Verification items for the finished model (mm, model axes). A direction names the side the tool comes from. Give positions to 0.01 mm unless a question says otherwise; leave off trailing zeros. Write each loop counter-clockwise with the first axis right and the second up, starting at its lowest first coordinate (ties: lowest second). Pieces come first, ordered by that corner, then holes. Notation, with made-up numbers: (-7, 89.25) -> (29, 89.25) arc R20 ccw to (29, 101.25) -> close; hole circle Ø1 at (-26.75, 72.25). An arc over 180 degrees is marked (long way). Write item = value, one per line.
from build123d import *

# Parameters (mm, degrees)
BOSS_EXTRUDE1_DEPTH = 3
SKETCH3_R           = 5.053902861
SKETCH3_R_2         = 2.749769833
BOSS_EXTRUDE3_DEPTH = 3
CUT_EXTRUDE1_DEPTH  = 3
SKETCH5_W           = 3
SKETCH5_H           = 8
CUT_EXTRUDE2_DEPTH  = 3


with BuildPart() as part:
    # Sketch1 → Boss-Extrude1 (new body)
    with BuildSketch(Plane.XY):
        with BuildLine():
            Line((-7, -3), (3, -3))
            Line((3, -3), (3, 0))
            Line((3, 0), (23, 0))
            Line((23, 0), (23, -3))
            Line((23, -3), (33, -3))
            Line((33, -3), (33, 0))
            Line((33, 0), (51.582575695, 0))
            ThreePointArc((51.582575695, 0), (51.894531565, 0.978451782), (52, 2))
            Line((52, 2), (52, 19.311841589))
            ThreePointArc((52, 19.311841589), (51.894531565, 20.333389808), (51.582575695, 21.311841589))
            Line((51.582575695, 21.311841589), (33, 21.311841589))
            Line((33, 21.311841589), (33, 24.311841589))
            Line((33, 24.311841589), (23, 24.311841589))
            Line((23, 24.311841589), (23, 21.311841589))
            Line((23, 21.311841589), (3, 21.311841589))
            Line((3, 21.311841589), (3, 24.311841589))
            Line((3, 24.311841589), (-7, 24.311841589))
            Line((-7, 24.311841589), (-7, 21.311841589))
            Line((-7, 21.311841589), (-25.582575695, 21.311841589))
            ThreePointArc((-25.582575695, 21.311841589), (-25.894531565, 20.333389808), (-26, 19.311841589))
            Line((-26, 19.311841589), (-26, 2))
            ThreePointArc((-26, 2), (-25.894531565, 0.978451782), (-25.582575695, 0))
            Line((-25.582575695, 0), (-7, 0))
            Line((-7, 0), (-7, -3))
        make_face()
    extrude(amount=BOSS_EXTRUDE1_DEPTH)

    # Sketch3 → Boss-Extrude3 (add)
    with BuildSketch(Plane(origin=(0, 0, 0), x_dir=(-1, 0, 0), z_dir=(0, 0, -1))):
        with Locations((20.946097139, 22.811841589)):
            Circle(SKETCH3_R)
        with Locations((20.946097139, 22.811841589)):
            Circle(SKETCH3_R_2, mode=Mode.SUBTRACT)
    extrude(amount=-BOSS_EXTRUDE3_DEPTH)

    # Sketch4 → Cut-Extrude1 (cut)
    with BuildSketch(Plane(origin=(0, 0, 0), x_dir=(-1, 0, 0), z_dir=(0, 0, -1))):
        with BuildLine():
            Line((23.250708633, 21.311841589), (18.641485645, 21.311841589))
            ThreePointArc((18.641485645, 21.311841589), (20.946097139, 20.062071756), (23.250708633, 21.311841589))
        make_face()
    extrude(amount=-CUT_EXTRUDE1_DEPTH, mode=Mode.SUBTRACT)

    # Sketch5 → Cut-Extrude2 (cut)
    with BuildSketch(Plane(origin=(0, 0, 0), x_dir=(-1, 0, 0), z_dir=(0, 0, -1))):
        with Locations((24.5, 10.655920795)):
            Rectangle(SKETCH5_W, SKETCH5_H)
        with Locations((-50.5, 10.655920795)):
            Rectangle(SKETCH5_W, SKETCH5_H)
    extrude(amount=-CUT_EXTRUDE2_DEPTH, mode=Mode.SUBTRACT)


solid = part.part
Item 1: Set-up check for faces 1 (the flat face through (51, 6.656, 1)), 2 (the flat face through (23, -1, 1)), 3 (the flat face through (-7, -1, 1)), 4 (the flat face through (42, 0, 1)): record each of +Z, -Z, +X, -X, +Y, -Y from which the full face is reachable in a straight line by a thin tool's end or side.
Response values:
face_1 = +Z, -Z, +X
face_2 = +Z, -Z, -Y
face_3 = +Z, -Z, -X, -Y
face_4 = +Z, -Z, +X, -Y
Item 2: Material ranges on line 1 (X direction, y = 22.5, z = 0.55); line 2 (Y direction, x = 29, z = 0.3); line 3 (Y direction, x = 35, z = 1.95), recorded low to high.
Response values:
line_1 = -25.99 to -23.68, -18.21 to -15.9, -7 to 3, 23 to 33
line_2 = -3 to 24.31
line_3 = 0 to 21.31
Item 3: Sectioned sample at A-A on x = 31.5. Record the cut outline in (y, z), then the cut area to 3 significant figures.
Response values:
outline = (-3, 0) -> (24.31, 0) -> (24.31, 3) -> (-3, 3) -> close
area = 81.9 mm^2
Item 4: Go/stop test with flat-tipped pins: P1, Ø1.5, axis at x = 17, z = 2, coming from the +Y side; P2, Ø0.9, axis at x = -17, z = 2, coming from the -Y side; P3, Ø1.5, axis at x = -24.5, z = 1, coming from the +Y side. Record where each tip stops, or that it passes through.
Response values:
P1 = 21.31
P2 = 0
P3 = 27.02
Item 5: Mould release check, pull along Y, two halves, no side actions. Record for faces 5 (the flat face through (-7, 23, 1)), 6 (the flat face through (-24, 6.656, 1)), 7 (the cylindrical face through (51.9, 20.3, 1.5)): +Y half, -Y half, draft (parallel to the pull), parting line (faces both ways), or undercut.
Response values:
face_5 = draft
face_6 = undercut
face_7 = +Y half
Item 6: Sectioned sample at B-B on y = 13. Record the cut outline in (x, z).
Response values:
outline = (-23, 0) -> (49, 0) -> (49, 3) -> (-23, 3) -> close
